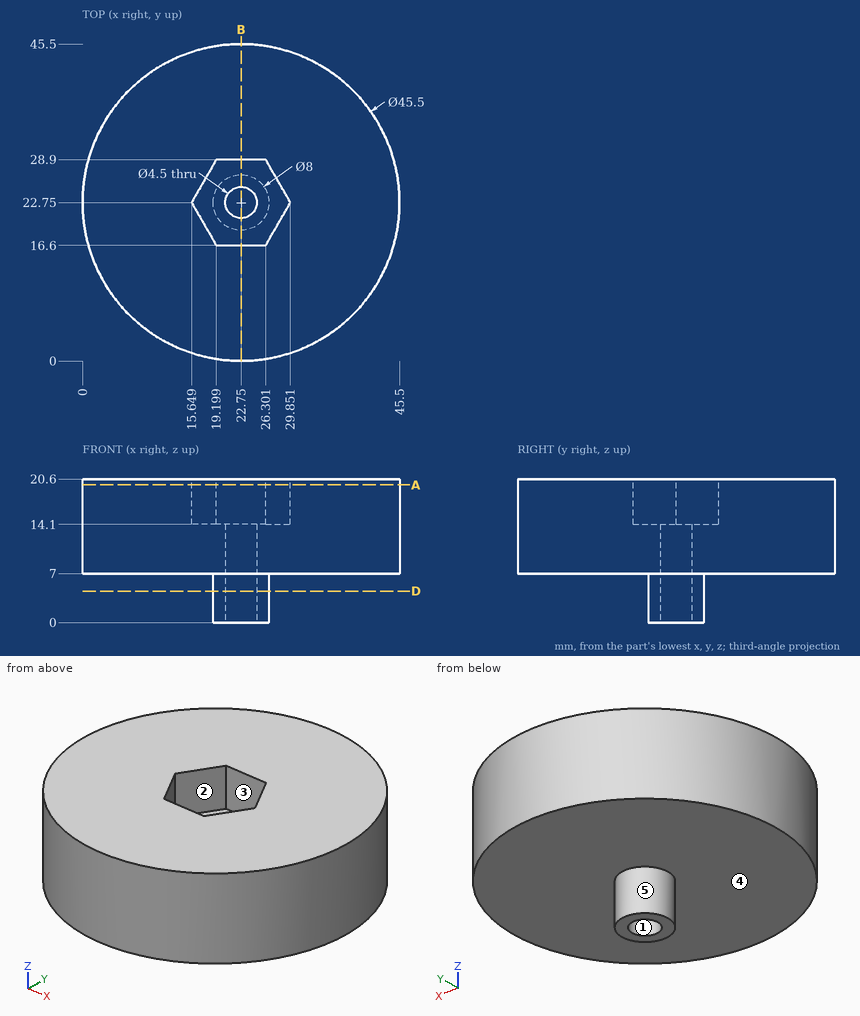
Input: dimensioned drawing with shaded views. Units: mm. Origin: part minimum x, y, z. A direction names the side the tool comes from. Coordinates: 2 decimals unless noted, no trailing zeros. Write each loop counter-clockwise with the first axis right and the second up, starting at its lowest first coordinate (ties: lowest second). Pieces come first, ordered by that corner, then holes. Notation, with made-up numbers: (-9.5, 81) -> (32.5, 81) arc R12 cw to (32.5, 101) -> close; hole circle Ø8 at (-22, 86.5). An arc over 180 degrees is marked (long way). Return JSON: item names as keys, results as strings. Group by question number.
1) Contact query for flat-ended pins moving along their axis: P1, Ø5, axis at x = 37, y = 16.5, coming from the -Z side; P2, Ø3.5, axis at x = 21.5, z = 18, coming from the -Y side; P3, Ø1, axis at y = 18, z = 14.5, coming from the -X side. Output: stop coordinate, or through.
2) Mould query, pull axis X, two halves, no side actions, for the marked faces 3, 4 and 5. Classes: +X half, -X half, draft (parallel to the pull), parting line (faces both ways), or undercut.
3) Set-up query: the marked faces 1 and 2. Return all of +Z, -Z, +X, -X, +Y, -Y with unobstructed straight access to the full face (end or side cutting, diameter ignored); none if empty.
4) Section query B-B, the plane x = 22.75. Return loops of the section in (y, z).
5) Section query D-D, the plane z = 4.5. Return loops of the section in (x, y).
6) Ray query, line 1 along Y through (x, z) = (22.75, 4); line 2 along Y through (x, z) = (22.75, 9.5); line 3 along Z through (x, y) = (40, 27.5). Return the intervals inside material, ascending.
7) Section query A-A, the plane z = 19.75. Return loops of the section in (x, y), plus the area to 4 significant figures.
From the geometry:
{
 "1": {"P1": "z = 7", "P2": "y = 0", "P3": "x = 0.4"},
 "2": {"face 3": "undercut", "face 4": "draft", "face 5": "parting line"},
 "3": {"face 1": "+Z, -Z", "face 2": "+Z"},
 "4": {"outline": "(0, 7) -> (18.75, 7) -> (18.75, 0) -> (20.5, 0) -> (20.5, 14.1) -> (16.6, 14.1) -> (16.6, 20.6) -> (0, 20.6) -> close; (25, 0) -> (26.75, 0) -> (26.75, 7) -> (45.5, 7) -> (45.5, 20.6) -> (28.9, 20.6) -> (28.9, 14.1) -> (25, 14.1) -> close"},
 "5": {"outline": "circle Ø8 at (22.75, 22.75); hole circle Ø4.5 at (22.75, 22.75)"},
 "6": {"line 1": "18.75 to 20.5, 25 to 26.75", "line 2": "0 to 20.5, 25 to 45.5", "line 3": "7 to 20.6"},
 "7": {"outline": "circle Ø45.5 at (22.75, 22.75); hole (15.65, 22.75) -> (19.2, 16.6) -> (26.3, 16.6) -> (29.85, 22.75) -> (26.3, 28.9) -> (19.2, 28.9) -> close", "area": "1,495 mm²"}
}
